The model under review builds one solid part; all positions refer to its coordinate system, in mm. A direction names the side the tool comes from. Round coordinates to 2 decimals unless told otherwise and drop trailing zeros. Write each loop counter-clockwise with the first axis right and the second up, starting at its lowest first coordinate (ties: lowest second). Pieces come first, ordered by that corner, then holes. Notation, with made-up numbers: (26, -4.75) - (56, -4.75) arc R25 cw to (56, 22.25) - close; hole circle Ø8 at (-11, -35.75). An arc over 180 degrees is marked (long way). Return JSON: item names as keys, results as strings.
from build123d import *

# Parameters (mm, degrees)
F0_R     = 35.9935602645
F1_DEPTH = 4
F3_W     = 31.1600742862
F3_H     = 3.6825519055
F3_H_2   = 3.9658267051
F4_DEPTH = 4.7
F6_DEPTH = 2


# Not quite as in the source:
# - a fillet or chamfer that OpenCascade refuses, or shapes differently, is made with other operations: its cross-section is extruded or revolved along the edge and cut away or added


with BuildPart() as f1:
    # F0 (on Top) → F1 (new body)
    with BuildSketch(Plane.XY):
        Circle(F0_R)
    extrude(amount=F1_DEPTH)

    # F2: fillet of radius 4.8284271247 on 1 edges, made by hand

    # F2_s1 → F2_t2 (revolve, cut)
    with BuildSketch(Plane.XZ):
        with BuildLine():
            ThreePointArc((35.9935602645, 0), (34.3442797526, 2.8670910053), (31.2367318045, 4))
            Line((31.2367318045, 4), (35.9935602645, 4))
            Line((35.9935602645, 4), (35.9935602645, 0))
        make_face()
    revolve(axis=Axis((0, 0, 4), (0, 0, 1)), mode=Mode.SUBTRACT)

    # F3 (on face) → F4 (join)
    with BuildSketch(Plane.XY.offset(4)):
        with Locations((1.6996399499, 19.9707737193)):
            Rectangle(F3_W, F3_H)
        with Locations((1.6996399499, -19.5458633825)):
            Rectangle(F3_W, F3_H_2)
    extrude(amount=F4_DEPTH)

    # F5 (on face) → F6 (cut)
    with BuildSketch(Plane(origin=(0, 0, 0), x_dir=(1, 0, 0), z_dir=(0, 0, -1))):
        with BuildLine():
            Line((1.0116308873, -10.4608191177), (4.1609390889, -1.4550810977))
            ThreePointArc((4.1609390889, -1.4550810977), (-0.0142907136, -4.4080007801), (-4.1702862527, -1.4280713123))
            Line((-4.1702862527, -1.4280713123), (-1.0771154127, -10.4608191177))
            Line((-1.0771154127, -10.4608191177), (-1.0116308873, -10.4608191177))
            ThreePointArc((-1.0116308873, -10.4608191177), (0, -9.4491882305), (1.0116308873, -10.4608191177))
        make_face()
        with BuildLine():
            ThreePointArc((-1.0116308873, -10.4608191177), (0, -11.472450005), (1.0116308873, -10.4608191177))
            Line((1.0116308873, -10.4608191177), (0, -10.4608191177))
            Line((0, -10.4608191177), (-1.0116308873, -10.4608191177))
        make_face()
        with BuildLine():
            Line((0, -10.4608191177), (1.0116308873, -10.4608191177))
            ThreePointArc((1.0116308873, -10.4608191177), (0, -9.4491882305), (-1.0116308873, -10.4608191177))
            Line((-1.0116308873, -10.4608191177), (0, -10.4608191177))
        make_face()
        with BuildLine():
            ThreePointArc((4.1609390889, -1.4550810977), (4.3458137466, -0.7379552708), (4.4080239453, 0))
            ThreePointArc((4.4080239453, 0), (0.7238623632, 4.3481833426), (-4.1702862527, 1.4280713123))
            ThreePointArc((-4.1702862527, 1.4280713123), (-4.4080239453, 0), (-4.1702862527, -1.4280713123))
            ThreePointArc((-4.1702862527, -1.4280713123), (-0.0142907136, -4.4080007801), (4.1609390889, -1.4550810977))
        make_face()
        with BuildLine():
            ThreePointArc((-4.1702862527, 1.4280713123), (0.7238623632, 4.3481833426), (4.4080239453, 0))
            ThreePointArc((4.4080239453, 0), (4.3458137466, -0.7379552708), (4.1609390889, -1.4550810977))
            Line((4.1609390889, -1.4550810977), (4.6697812098, 0))
            Line((4.6697812098, 0), (1.0316451427, 10.5936024338))
            ThreePointArc((1.0316451427, 10.5936024338), (0, 9.5619572911), (-1.0316451427, 10.5936024338))
            Line((-1.0316451427, 10.5936024338), (-4.1702862527, 1.4280713123))
        make_face()
        with BuildLine():
            ThreePointArc((1.0316451427, 10.5936024338), (0, 11.6252475765), (-1.0316451427, 10.5936024338))
            Line((-1.0316451427, 10.5936024338), (0, 10.5936024338))
            Line((0, 10.5936024338), (1.0316451427, 10.5936024338))
        make_face()
        with BuildLine():
            Line((0, 10.5936024338), (-1.0316451427, 10.5936024338))
            ThreePointArc((-1.0316451427, 10.5936024338), (0, 9.5619572911), (1.0316451427, 10.5936024338))
            Line((1.0316451427, 10.5936024338), (0, 10.5936024338))
        make_face()
    extrude(amount=-F6_DEPTH, mode=Mode.SUBTRACT)


solid = f1.part
(1) Clearance check with flat-ended pins moving along their axes: pin 1 Ø5 at (x, z) = (1.5, 6) entering from +Y; pin 2 Ø1.4 at (x, z) = (7, 7.5) entering from -Y; pin 3 Ø1.8 at (y, z) = (20.5, 5.5) entering from +X. State where each tip first meets the part, or that it passes through.
Filled in:
{"pin 1": "stops at y = 33.34", "pin 2": "stops at y = -21.53", "pin 3": "stops at x = 17.28"}
(2) Add section A-A (z = 7.5). Write out the cut boundary in (x, y), plus the area to 3 significant figures.
Filled in:
{"outline": "(-13.88, -21.53) - (17.28, -21.53) - (17.28, -17.56) - (-13.88, -17.56) - close; (-13.88, 18.13) - (17.28, 18.13) - (17.28, 21.81) - (-13.88, 21.81) - close", "area": "238 mm2"}
(3) For faces 1 (the flat face through (-2.645, 5.881, 0.986)), 2 (the flat face through (-13.88, 20, 6)), 3 (the flat face through (1, 18.129, 6)), 4 (the flat face through (1, 21.812, 6)), list the 3-axis set-ups (+Z, -Z, +X, -X, +Y, -Y) from which the entire face can be reached by the end or side of a thin tool; tool diameter is ignored.
Filled in:
{"face 1": "-Z", "face 2": "+Z, -X, +Y, -Y", "face 3": "+Z, +X, -X", "face 4": "+Z, +X, -X, +Y"}
(4) Wall thickness on line 1 (Y direction, x = -13.5, z = 4.5); line 2 (Z direction, x = 2.5, y = 12.5); line 3 (X direction, y = -18.5, z = 7.75): over which ranges is each line inside the solid? List them lowest first.
Filled in:
{"line 1": "y = -21.53 to -17.56, 18.13 to 21.81", "line 2": "z = 0 to 4", "line 3": "x = -13.88 to 17.28"}
(5) Mouldability with a two-part tool opening along X and no side actions: class faces 5 (the flat face through (-13.88, -20, 6)), 6 (the flat face through (17.28, 20, 6)), 7 (the cylindrical face through (-4.408, -0.02, 0.986)) as released by +X, released by -X, zero draft, split by the parting line, or undercut.
Filled in:
{"face 5": "released by -X", "face 6": "released by +X", "face 7": "undercut"}
(6) Add section B-B (x = 0). Write out the cut boundary in (y, z).
Filled in:
{"outline": "(-35.99, 0) - (-11.63, 0) - (-11.63, 2) - (11.47, 2) - (11.47, 0) - (35.99, 0) arc R4.83 ccw to (31.24, 4) - (21.81, 4) - (21.81, 8.7) - (18.13, 8.7) - (18.13, 4) - (-17.56, 4) - (-17.56, 8.7) - (-21.53, 8.7) - (-21.53, 4) - (-31.24, 4) arc R4.83 ccw to start"}
